Source: CAD feature listing. Evaluate the final solid. Frame: model axes, mm. A direction names the side the tool comes from. Give positions to 0.01 mm unless a question says otherwise; leave off trailing zeros. Order: outer loops, then holes, each group sorted by start corner. A loop starts at its lowest first (then second) coordinate and runs counter-clockwise, first axis right, second up. Notation, with made-up numbers: M 85.5,85 L 133.5,85 A8 ccw 133.5,95 Z; hole C 29.5,43.25 d3. An arc over 180 degrees is marked long. Use CSV: the item, a comma, the result in double quotes. Start each with the question number.
1. Pin query (flat end, axial travel): P1, Ø2, axis at x = -13, z = 123.5, coming from the -Y side; P2, Ø4, axis at y = -22, z = 147, coming from the -X side; P3, Ø4, axis at x = -17.5, y = 12, coming from the +Z side (3 decimals). Return the tip coordinate at first contact, or that it passes through.
2. Section query A-A, the plane y = 0. Return the cut outline in (x, z) (3 decimals).
3. Line query: line 1 along X through (y, z) = (0, 177) (3 decimals); line 2 along X through (y, z) = (0, 175.7) (3 decimals); line 3 along X through (y, z) = (0, 175) (3 decimals). Output: solid intervals per line, ascending. Write a range as [from, to].
4. Mould query, pull axis Z, two halves, no side actions, for faces 1 (the cylindrical face through (-81.596, -10.713, 176.512)), 2 (the cylindrical face through (80.96, -17.98, 175.91)), 3 (the flat face through (-1, 1, 0)). Classes: released by +Z, released by -Z, zero draft, split by the parting line, or undercut.
5. Reachability of faces 4 (the cylindrical face through (-82.477, -10.829, 87.664)), 5 (the cylindrical face through (-83.107, -10.912, 89.114)), 6 (the cylindrical face through (69.43, -15.42, 176.19)), 7 (the flat face through (-69.4, -16.3, 177.8)) from +Z, -Z, +X, -X, +Y, -Y: full face, straight path, thin tool, end or side. Return the list, or none.
6. Section query C-C, the plane z = 158. Return the cut outline in (x, y) (3 decimals).
from build123d import *


with BuildPart() as f1:
    # F0 (on Right) → F1 (revolve)
    with BuildSketch(Plane.YZ):
        with BuildLine():
            Line((0, 0.635), (0, 0))
            Line((0, 0), (83.82, 0))
            Line((83.82, 0), (83.82, 175.768))
            ThreePointArc((83.82, 175.768), (84.836, 176.784), (83.82, 177.8))
            Line((83.82, 177.8), (82.296, 177.8))
            Line((82.296, 177.8), (82.296, 175.26))
            Line((82.296, 175.26), (71.755, 175.26))
            Line((71.755, 175.26), (71.755, 177.8))
            Line((71.755, 177.8), (71.12, 177.8))
            Line((71.12, 177.8), (71.12, 174.625))
            Line((71.12, 174.625), (82.931, 174.625))
            Line((82.931, 174.625), (82.931, 177.165))
            Line((82.931, 177.165), (83.185, 177.165))
            Line((83.185, 177.165), (83.185, 0.635))
            Line((83.185, 0.635), (0, 0.635))
        make_face()
    revolve(axis=Axis((0, 0, 48.229507), (0, 0, 1)))


solid = f1.part
Result set:
1,P1,"y = -82.96"
1,P2,"x = -81.4"
1,P3,"z = 0.635"
2,outline,"M -83.82,0 L 83.82,0 L 83.82,175.768 A1.016 ccw 83.82,177.8 L 82.296,177.8 L 82.296,175.26 L 71.755,175.26 L 71.755,177.8 L 71.12,177.8 L 71.12,174.625 L 82.931,174.625 L 82.931,177.165 L 83.185,177.165 L 83.185,0.635 L -83.185,0.635 L -83.185,177.165 L -82.931,177.165 L -82.931,174.625 L -71.12,174.625 L -71.12,177.8 L -71.755,177.8 L -71.755,175.26 L -82.296,175.26 L -82.296,177.8 L -83.82,177.8 A1.016 ccw -83.82,175.768 Z"
3,line 1,"[-84.813, -83.185], [-82.931, -82.296], [-71.755, -71.12], [71.12, 71.755], [82.296, 82.931], [83.185, 84.813]"
3,line 2,"[-83.82, -83.185], [-82.931, -82.296], [-71.755, -71.12], [71.12, 71.755], [82.296, 82.931], [83.185, 83.82]"
3,line 3,"[-83.82, -83.185], [-82.931, -71.12], [71.12, 82.931], [83.185, 83.82]"
4,face 1,"zero draft"
4,face 2,"undercut"
4,face 3,"released by -Z"
5,face 4,"none"
5,face 5,"-Z"
5,face 6,"+Z"
5,face 7,"+Z, +X, -X, +Y, -Y"
6,outline,"C 0,0 d167.64; hole C 0,0 d166.37"
